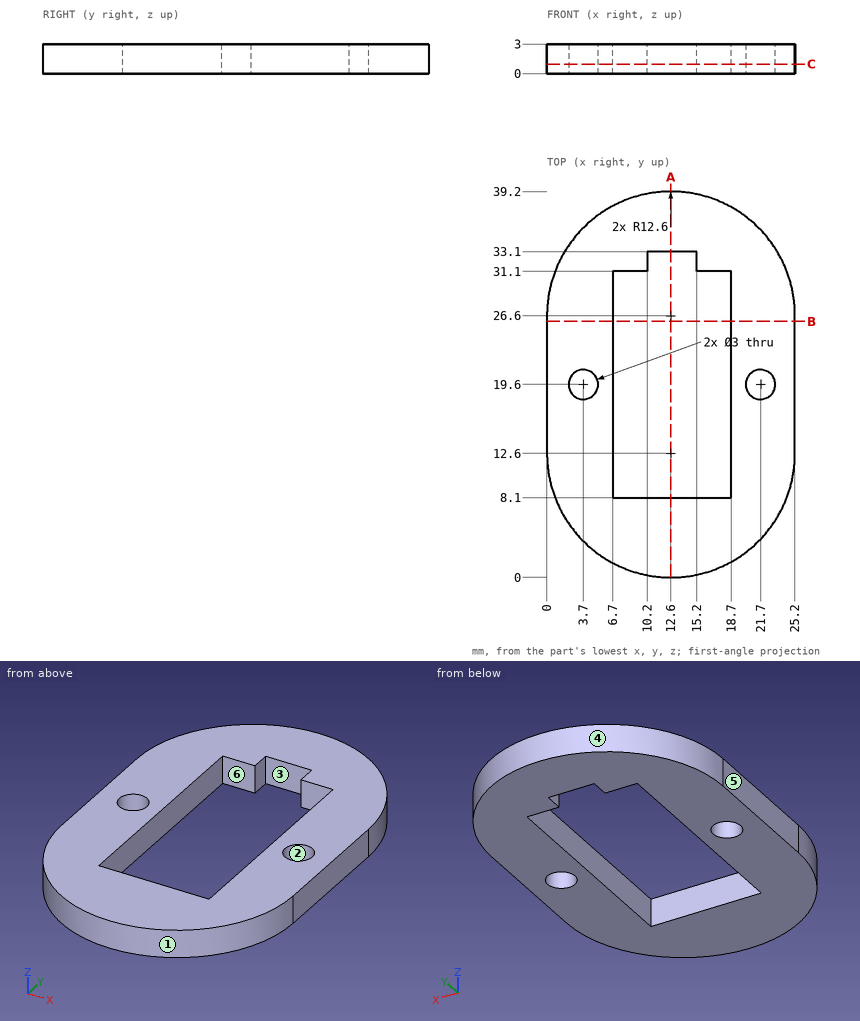
Print and shaded views of the part. All mm, measured from the part's lowest x, y and z. A direction names the side the tool comes from. Round coordinates to 2 decimals unless told otherwise and drop trailing zeros. Write each loop counter-clockwise with the first axis right and the second up, starting at its lowest first coordinate (ties: lowest second). Pieces come first, ordered by that corner, then holes. Notation, with made-up numbers: (-35.5, -37.5) -> (8.5, -37.5) arc R23 ccw to (8.5, -15.5) -> close; hole circle Ø1 at (45.25, -7.75). An arc over 180 degrees is marked (long way). Return JSON: item names as keys, results as strings. Group by question number.
Q1. Mould opens along Y. For the marked faces 1, 2, 3 and 4 say: pulls with the +Y half, pulls with the -Y half, needs draft (parallel to the pull), parting line crosses it, or undercut.
Q2. Saw through at A-A on x = 12.6. Write the cut outline in (y, z).
Q3. Saw through at C-C on z = 0.95. Write the cut outline in (x, y).
Q4. Probe L1, parallel to X at y = 24, z = 1.6; L2, parallel to Y at x = 3.25, z = 2.4; L3, parallel to Y at x = 4.5, z = 1.7. List the from-to ranges inside material, lowest first. Write a range as [from, to].
Q5. Saw through at B-B on y = 26. Write the cut outline in (x, z).
Q6. Which spindle directions (+Z, -Z, +X, -X, +Y, -Y) get a long thin tool onto all of the face, cutting with end or side? Do the marked faces 5 and 6. Say none if no direction does.
Q7. Pin check, flat tips, straight feed: pin 1 (2.5 mm diameter, centred on x = 3.7, y = 19.6, fed in from -Z); pin 2 (0.9 mm diameter, centred on x = 11.5, z = 2, fed in from +Y); pin 3 (0.6 mm diameter, centred on y = 32.5, z = 1.5, fed in from +X); pin 4 (1.6 mm diameter, centred on y = 32, z = 2, fed in from -X). Stop position of each tip, or through.
Answer:
{
 "1": {"face 1": "pulls with the -Y half", "face 2": "undercut", "face 3": "undercut", "face 4": "pulls with the +Y half"},
 "2": {"outline": "(0, 0) -> (8.1, 0) -> (8.1, 3) -> (0, 3) -> close; (33.1, 0) -> (39.2, 0) -> (39.2, 3) -> (33.1, 3) -> close"},
 "3": {"outline": "(0, 12.6) arc R12.6 ccw to (25.2, 12.6) -> (25.2, 26.6) arc R12.6 ccw to (0, 26.6) -> close; hole circle Ø3 at (3.7, 19.6); hole (6.7, 8.1) -> (18.7, 8.1) -> (18.7, 31.1) -> (15.2, 31.1) -> (15.2, 33.1) -> (10.2, 33.1) -> (10.2, 31.1) -> (6.7, 31.1) -> close; hole circle Ø3 at (21.7, 19.6)"},
 "4": {"L1": "[0, 6.7], [18.7, 25.2]", "L2": "[4.15, 18.17], [21.03, 35.05]", "L3": "[2.95, 18.33], [20.87, 36.25]"},
 "5": {"outline": "(0, 0) -> (6.7, 0) -> (6.7, 3) -> (0, 3) -> close; (18.7, 0) -> (25.2, 0) -> (25.2, 3) -> (18.7, 3) -> close"},
 "6": {"face 5": "+Z, -Z, -X, +Y, -Y", "face 6": "+Z, -Z"},
 "7": {"pin 1": "through", "pin 2": "y = 39.18", "pin 3": "x = 23.89", "pin 4": "x = 0.87"}
}
